from build123d import *

# Parameters (mm, degrees)
SKETCH1_R           = 76
SKETCH1_R_2         = 1.5
BOSS_EXTRUDE1_DEPTH = 50
CUT_EXTRUDE1_START  = -40
CUT_EXTRUDE1_DEPTH  = 40


with BuildPart() as part:
    # Sketch1 → Boss-Extrude1 (new body)
    with BuildSketch(Plane.XY):
        Polygon((103.923048454, 0), (51.961524227, 90), (-51.961524227, 90), (-103.923048454, 0), (-51.961524227, -90), (51.961524227, -90), align=None)
        Circle(SKETCH1_R, mode=Mode.SUBTRACT)
        with Locations((30, -85)):
            Circle(SKETCH1_R_2, mode=Mode.SUBTRACT)
        with Locations((-30, -85)):
            Circle(SKETCH1_R_2, mode=Mode.SUBTRACT)
        with Locations((30, 85)):
            Circle(SKETCH1_R_2, mode=Mode.SUBTRACT)
        with Locations((-30, 85)):
            Circle(SKETCH1_R_2, mode=Mode.SUBTRACT)
    extrude(amount=BOSS_EXTRUDE1_DEPTH)

    # Sketch4 → Cut-Extrude1 (cut)
    with BuildSketch(Plane.XY.offset(50).offset(CUT_EXTRUDE1_START)):
        with BuildLine():
            ThreePointArc((68.461668107, 33), (74.091452868, 16.925029156), (76, 0))
            Line((76, 0), (103.923048454, 0))
            Line((103.923048454, 0), (84.870489571, 33))
            Line((84.870489571, 33), (68.461668107, 33))
        make_face()
        with BuildLine():
            Line((103.923048454, 0), (76, 0))
            ThreePointArc((76, 0), (74.091452868, -16.925029156), (68.461668107, -33))
            Line((68.461668107, -33), (84.870489571, -33))
            Line((84.870489571, -33), (103.923048454, 0))
        make_face()
    extrude(amount=CUT_EXTRUDE1_DEPTH, mode=Mode.SUBTRACT)


solid = part.part
Design review of the part built by this model. Coordinates are the model's own, in mm. A direction names the side the tool comes from. Coordinates: 2 decimals unless noted, no trailing zeros. Loops run counter-clockwise (first coordinate to the right, second up) from the corner with the lowest first, then second, coordinate; pieces in that order, holes last.
Item 1: Wall thickness on L1, parallel to X at y = 85, z = 12; L2, parallel to Y at x = -30, z = 34; L3, parallel to Z at x = 84.5, y = -30: over which ranges is each line inside the solid? List them lowest first.
Completed:
L1: x = -54.85 to -31.5, -28.5 to 28.5, 31.5 to 54.85
L2: y = -90 to -86.5, -83.5 to -69.83, 69.83 to 83.5, 86.5 to 90
L3: z = 0 to 10
Item 2: Add section B-B (x = 0). Write out the cut boundary in (y, z), and give its area (3 significant figures).
Completed:
outline: (-90, 0) - (-76, 0) - (-76, 50) - (-90, 50) - close; (76, 0) - (90, 0) - (90, 50) - (76, 50) - close
area: 1,400 mm2
Item 3: Draft analysis for pull direction Y (two halves, no side actions). For faces 1 (the flat face through (1, 90, 25)), 2 (the flat face through (-1, -90, 25)), 3 (the flat face through (61, -46, 0)), 4 (the cylindrical face through (-75.927, 3.342, 24.65)), state which applies: pulls with the +Y half, pulls with the -Y half, needs draft (parallel to the pull), parting line crosses it, or undercut.
Completed:
face 1: pulls with the +Y half
face 2: pulls with the -Y half
face 3: needs draft
face 4: undercut
Item 4: Add section D-D (z = 21). Write out the cut boundary in (x, y), and give its area (3 significant figures).
Completed:
outline: (-103.92, 0) - (-51.96, -90) - (51.96, -90) - (84.87, -33) - (68.46, -33) arc R76 cw (long way) to (68.46, 33) - (84.87, 33) - (51.96, 90) - (-51.96, 90) - close; hole circle Ø3 at (-30, -85); hole circle Ø3 at (-30, 85); hole circle Ø3 at (30, -85); hole circle Ø3 at (30, 85)
area: 8,510 mm2
Item 5: Add section A-A (z = 6). Write out the cut boundary in (x, y), and give its area (3 significant figures).
Completed:
outline: (-103.92, 0) - (-51.96, -90) - (51.96, -90) - (103.92, 0) - (51.96, 90) - (-51.96, 90) - close; hole circle Ø152 at (0, 0); hole circle Ø3 at (-30, -85); hole circle Ø3 at (-30, 85); hole circle Ø3 at (30, -85); hole circle Ø3 at (30, 85)
area: 9,890 mm2
Item 6: Clearance check with flat-ended pins moving along their axes: pin 1 (4 mm diameter, centred on y = -4, z = 33, fed in from +X); pin 2 (5 mm diameter, centred on x = 78, z = 20, fed in from +Y); pin 3 (10.5 mm diameter, centred on x = 83, y = 16, fed in from +Z); pin 4 (2.5 mm diameter, centred on x = -30, y = 85, fed in from +Z). State where each tip first meets the part, or that it passes through.
Completed:
pin 1: stops at x = -75.76
pin 2: stops at y = 49.23
pin 3: stops at z = 10
pin 4: passes through
Item 7: Add section C-C (y = 49.5). Write out the cut boundary in (x, z), and give its area (3 significant figures).
Completed:
outline: (-75.34, 0) - (-57.67, 0) - (-57.67, 50) - (-75.34, 50) - close; (57.67, 0) - (75.34, 0) - (75.34, 50) - (57.67, 50) - close
area: 1,770 mm2
Item 8: For faces 5 (the flat face through (-73, 27, 50)), 6 (the flat face through (77, 33, 30)), list the 3-axis set-ups (+Z, -Z, +X, -X, +Y, -Y) from which the entire face can be reached by the end or side of a thin tool; tool diameter is ignored.
Completed:
face 5: +Z, +X, -X, +Y, -Y
face 6: +Z, +X
